from build123d import *

# Parameters (mm, degrees)
SKETCH1_W                        = 41
SKETCH1_H                        = 70
BOSS_EXTRUDE1_DEPTH              = 25
CUT_EXTRUDE1_DEPTH               = 16
TAP_DRILL_FOR_M16X2_0_TAP1_D     = 14
TAP_DRILL_FOR_M16X2_0_TAP1_DEPTH = 24.377223398
TAP_DRILL_FOR_M16X2_0_TAP1_TIP   = 4.206024333
FILLET1_R                        = 10
FILLET2_R                        = 0.9
FILLET4_R                        = 5


with BuildPart() as part:
    # Sketch1 → Boss-Extrude1 (new body)
    with BuildSketch(Plane.XY):
        Rectangle(SKETCH1_W, SKETCH1_H)
    extrude(amount=BOSS_EXTRUDE1_DEPTH)

    # Sketch6 → Cut-Extrude1 (cut)
    with BuildSketch(Plane.XY.offset(25)):
        with BuildLine():
            Line((-3.6, -35), (-3.6, -33))
            ThreePointArc((-3.6, -33), (-5.694183484, -19.431989494), (-11.781818182, -7.126819144))
            ThreePointArc((-11.781818182, -7.126819144), (-13.134625892, -4.392336844), (-13.6, -1.377223398))
            Line((-13.6, -1.377223398), (-13.6, 3.622776602))
            Line((-13.6, 3.622776602), (13.6, 3.622776602))
            Line((13.6, 3.622776602), (13.6, -1.377223398))
            ThreePointArc((13.6, -1.377223398), (13.134625892, -4.392336844), (11.781818182, -7.126819144))
            ThreePointArc((11.781818182, -7.126819144), (5.694183484, -19.431989494), (3.6, -33))
            Line((3.6, -33), (3.6, -35))
            Line((3.6, -35), (-3.6, -35))
        make_face()
    extrude(amount=-CUT_EXTRUDE1_DEPTH, mode=Mode.SUBTRACT)

    # Tap Drill for M16x2.0 Tap1
    with Locations(Plane(origin=(0, 35, 0), x_dir=(1, 0, 0), z_dir=(0, 1, 0))):
        with Locations((0, -12.5)):
            Hole(TAP_DRILL_FOR_M16X2_0_TAP1_D / 2, depth=TAP_DRILL_FOR_M16X2_0_TAP1_DEPTH)
            with Locations((0, 0, -(TAP_DRILL_FOR_M16X2_0_TAP1_DEPTH + TAP_DRILL_FOR_M16X2_0_TAP1_TIP / 2))):  # 118° drill point
                Cone(0, TAP_DRILL_FOR_M16X2_0_TAP1_D / 2, TAP_DRILL_FOR_M16X2_0_TAP1_TIP, mode=Mode.SUBTRACT)

    # Fillet1
    fillet1_edges = [part.edges().sort_by_distance(p)[0] for p in [
        (20.5, -35, 12.5),
        (-20.5, -35, 12.5),
        (-20.5, 35, 12.5),
        (20.5, 35, 12.5),
    ]]
    fillet(fillet1_edges, radius=FILLET1_R)

    # Fillet2
    fillet2_edges = [part.edges().sort_by_distance(p)[0] for p in [
        (-13.6, 3.622776602, 17),
        (13.6, 3.622776602, 17),
    ]]
    fillet(fillet2_edges, radius=FILLET2_R)

    # Fillet4
    # the kernel refuses this fillet: 5 mm, written as the material it takes off along each edge
    with BuildSketch(Plane(origin=(3.6, -35, 38.441235127), x_dir=(1, 0, 0), z_dir=(0, 0, -1))) as fillet4_piece_1:
        with BuildLine():
            CenterArc((5.11265865, -5), FILLET4_R, 90, 94.301222305)
            Line((0.126740981, -5.375), (-0.371850786, -5.4125))
            ThreePointArc((-0.371850786, -5.4125), (-0.5, -2), (-0.5, 0))
            Line((-0.5, 0), (0, 0.5))
            Line((0, 0.5), (5.11265865, 0.5))
            Line((5.11265865, 0.5), (5.11265865, 0))
        make_face()
    extrude(amount=29.441235127, mode=Mode.SUBTRACT)
    with BuildSketch(Plane(origin=(-3.6, -35, 38.441235127), x_dir=(-0.0235731649015064, 0.9997221143380427, 0), z_dir=(0, 0, -1))) as fillet4_piece_2:
        with BuildLine():
            CenterArc((5.119132117, -4.993372091), FILLET4_R, 87.049545676, 94.301222305)
            Line((0.120521545, -5.111237915), (-0.379339512, -5.123024498))
            Line((-0.379339512, -5.123024498), (-0.499861057, -0.011786582))
            Line((-0.499861057, -0.011786582), (-0.011786582, 0.499861057))
            ThreePointArc((-0.011786582, 0.499861057), (1.987657646, 0.547007387), (5.402230244, 0.499337209))
            Line((5.402230244, 0.499337209), (5.376494051, 0))
        make_face()
    extrude(amount=29.441235127, mode=Mode.SUBTRACT)


solid = part.part
CAD build for the part. Positions are in the model's coordinates, mm. A direction names the side the tool comes from. Round coordinates to 2 decimals unless told otherwise and drop trailing zeros. Order: outer loops, then holes, each group sorted by start corner. A loop starts at its lowest first (then second) coordinate and runs counter-clockwise, first axis right, second up. Notation, with made-up numbers: M 74,21 L 118,21 A26 ccw 118,38 Z; hole C -1.5,26.5 d11. An arc over 180 degrees is marked long. Use one line per item in the form item = value.
Q1. Probe L1, parallel to Z at x = 0, y = 21.5; L2, parallel to X at y = -1, z = 23.5; L3, parallel to Z at x = 2.5, y = 17. List the from-to ranges inside material, lowest first.
Recorded:
L1 = 0 to 5.5, 19.5 to 25
L2 = -20.5 to -13.6, 13.6 to 20.5
L3 = 0 to 5.96, 19.04 to 25
Q2. Two-plate mould, pull along Z, no slides. Class faces 3 (the flat face through (-13.6, 1, 17)), 4 (the cylindrical face through (1.517, 22.641, 19.334)), 5 (the flat face through (0, 8, 25)): +Z half, -Z half, draft (parallel to the pull), parting line (faces both ways), or undercut.
Recorded:
face_3 = draft
face_4 = undercut
face_5 = +Z half
Q3. Saw through at A-A on z = 20.25. Give the cut face in (x, y) (3 decimals).
Recorded:
outline = M -20.5,-25 A10 ccw -10.5,-35 L -8.713,-35 A5 ccw -3.727,-29.625 A45 ccw -11.782,-7.127 A10 cw -13.6,-1.377 L -13.6,2.723 A0.9 cw -12.7,3.623 L 12.7,3.623 A0.9 cw 13.6,2.723 L 13.6,-1.377 A10 cw 11.782,-7.127 A45 ccw 3.727,-29.625 A5 ccw 8.713,-35 L 10.5,-35 A10 ccw 20.5,-25 L 20.5,25 A10 ccw 10.5,35 L -10.5,35 A10 ccw -20.5,25 Z
Q4. Saw through at B-B on y = 0. Give the cut face in (x, z), then the cut area to 3 significant figures.
Recorded:
outline = M -20.5,0 L 20.5,0 L 20.5,25 L 13.6,25 L 13.6,9 L -13.6,9 L -13.6,25 L -20.5,25 Z
area = 590 mm^2
Q5. Saw through at C-C on x = -16.5. Give the cut face in (y, z), then the cut area to 3 significant figures.
Recorded:
outline = M -33,0 L 33,0 L 33,25 L -33,25 Z
area = 1,650 mm^2
Q6. Which spindle directions (+Z, -Z, +X, -X, +Y, -Y) get a long thin tool onto all of the face, cutting with end or side? Do faces 1 (the flat face through (0, 3.623, 17)), 2 (the flat face through (0, 0, 0)). Say none if no direction does.
Recorded:
face_1 = +Z
face_2 = -Z, +X, -X, +Y, -Y
Q7. Saw through at D-D on z = 2. Give the cut face in (x, y), then the cut area to 3 significant figures.
Recorded:
outline = M -20.5,-25 A10 ccw -10.5,-35 L 10.5,-35 A10 ccw 20.5,-25 L 20.5,25 A10 ccw 10.5,35 L -10.5,35 A10 ccw -20.5,25 Z
area = 2,780 mm^2
